Can you work these out from the model? Positions are in its coordinate system, mm. Face numbers are marked on the shaded views. Give positions to 0.01 mm unless a question says otherwise; leave off trailing zeros. Loops run counter-clockwise (first coordinate to the right, second up) from the corner with the lowest first, then second, coordinate; pieces in that order, holes last. Notation, with made-up numbers: (47.5, 39.25) - (51.5, 39.25) arc R18 ccw to (51.5, 61.25) - close; hole circle Ø3 at (17, 9). An arc over 180 degrees is marked (long way). Answer in a Markdown table with one row per item.
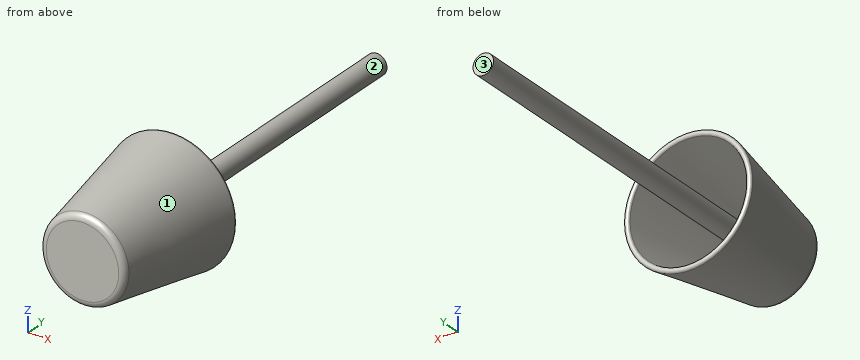
from build123d import *

# Parameters (mm, degrees)
ESQUISSE1_R        = 12.5
BOSS_EXTRU_2_DEPTH = 500


with BuildPart() as part:
    # Sketch1 → Revolve1 (revolve)
    with BuildSketch(Plane.XY):
        with BuildLine():
            Line((0, 0), (44.139646678, 0))
            ThreePointArc((44.139646678, 0), (49.241773329, 1.857022233), (51.956558217, 6.55916759))
            Line((51.956558217, 6.55916759), (77.67223186, 152.4))
            ThreePointArc((77.67223186, 152.4), (74.751767132, 155.587127984), (71.32223186, 152.955553013))
            Line((71.32223186, 152.955553013), (45.703028985, 7.661833518))
            ThreePointArc((45.703028985, 7.661833518), (45.160072008, 6.721404447), (44.139646678, 6.35))
            Line((44.139646678, 6.35), (0, 6.35))
            Line((0, 6.35), (0, 0))
        make_face()
    revolve(axis=Axis((0, 0, 0), (0, 1, 0)))

    # Esquisse1 → Boss.-Extru.2 (add)
    with BuildSketch(Plane(origin=(0, 6.35, 0), x_dir=(1, 0, 0), z_dir=(0, 1, 0))):
        Circle(ESQUISSE1_R)
    extrude(amount=BOSS_EXTRU_2_DEPTH)


solid = part.part
Q1. If we mould it in two halves opening along Z, with no side actions, what happens to the marked faces 1, 2 and 3? For each: released by +Z, released by -Z, zero draft, split by the parting line, or undercut.
Checked values:
| item | result |
|---|---|
| face 1 | split by the parting line |
| face 2 | undercut |
| face 3 | zero draft |
Q2. Imagine slicing it at C-C, the plane y = 310. Write out the boundary of the cut face in (x, z), and give its area (3 significant figures).
Checked values:
| item | result |
|---|---|
| outline | circle Ø25 at (0, 0) |
| area | 491 mm² |
Q3. For pin 1 (1.5 mm diameter, centred on y = 307, z = -0.5, fed in from -X); pin 2 (2 mm diameter, centred on x = 54, y = 147, fed in from +Z); pin 3 (8 mm diameter, centred on x = 8, y = 331.5, fed in from -Z), each with a flat end and sliding along its axis, tell me the tip position at first contact or that it passes through.
Checked values:
| item | result |
|---|---|
| pin 1 | stops at x = -12.5 |
| pin 2 | stops at z = 55.5 |
| pin 3 | stops at z = -11.84 |
Q4. If I drill on line 1 (X direction, y = 26, z = -9); line 2 (Y direction, x = -14, z = 1); line 3 (Z direction, x = -28, y = 38), over which ranges is the centre line in solid material (lowest first)? Write a range as [from, to].
Checked values:
| item | result |
|---|---|
| line 1 | x = [-54.65, -48.1], [-8.67, 8.67], [48.1, 54.65] |
| line 2 | y = [0, 6.35] |
| line 3 | z = [-50.22, -42.69], [42.69, 50.22] |
